```python
from build123d import *

# Parameters (mm, degrees)
SKETCH1_W               = 25.4
SKETCH1_H               = 17.78
BOSS_EXTRUDE1_DEPTH     = 1.6002
CUT_EXTRUDE1_DEPTH      = 16.584695699
CUT_EXTRUDE1_DEPTH_BACK = 16.584695699
SKETCH2_R               = 1.5875
SKETCH3_W               = 15.24
SKETCH3_H               = 2.54
BOSS_EXTRUDE2_DEPTH     = 2.54
SKETCH4_R               = 0.4064
BOSS_EXTRUDE3_DEPTH     = 5.969
LPATTERN1_COUNT         = 6
LPATTERN1_PITCH         = 2.54
MIRROR1_COPY_1_SKETCH_R = 0.4064
MIRROR1_COPY_1_DEPTH    = 5.969
MIRROR1_COPY_2_SKETCH_R = 0.4064
MIRROR1_COPY_2_DEPTH    = 5.969
MIRROR1_COPY_3_SKETCH_R = 0.4064
MIRROR1_COPY_3_DEPTH    = 5.969
MIRROR1_COPY_4_SKETCH_R = 0.4064
MIRROR1_COPY_4_DEPTH    = 5.969
MIRROR1_COPY_5_SKETCH_R = 0.4064
MIRROR1_COPY_5_DEPTH    = 5.969
SKETCH5_W               = 4.445
SKETCH5_H               = 6.35
BOSS_EXTRUDE4_DEPTH     = 3.175


with BuildPart() as part:
    # Sketch1 → Boss-Extrude1 (new body)
    with BuildSketch(Plane(origin=(0, 0, 0), x_dir=(1, 0, 0), z_dir=(0, 1, 0))):
        Rectangle(SKETCH1_W, SKETCH1_H)
    extrude(amount=BOSS_EXTRUDE1_DEPTH)

    # Sketch2 → Cut-Extrude1 (cut, two sides: drawn at the far end of the back side and taken through both)
    with BuildSketch(Plane(origin=(0, 1.6002, 0), x_dir=(1, 0, 0), z_dir=(0, 1, 0)).offset(-CUT_EXTRUDE1_DEPTH_BACK)):
        with Locations(Location((-10.16, 6.35, 0), (0, 0, 270))):
            Circle(SKETCH2_R)
        with Locations(Location((10.16, 6.35, 0), (0, 0, 270))):
            Circle(SKETCH2_R)
        with Locations(Location((10.16, -6.35, 0), (0, 0, 270))):
            Circle(SKETCH2_R)
        with Locations(Location((-10.16, -6.35, 0), (0, 0, 270))):
            Circle(SKETCH2_R)
        with BuildLine():
            Line((-12.7, 6.35), (-12.7, 8.89))
            Line((-12.7, 8.89), (-10.16, 8.89))
            ThreePointArc((-10.16, 8.89), (-11.956051224, 8.146051224), (-12.7, 6.35))
        make_face()
        with BuildLine():
            Line((10.16, 8.89), (12.7, 8.89))
            Line((12.7, 8.89), (12.7, 6.35))
            ThreePointArc((12.7, 6.35), (11.956051224, 8.146051224), (10.16, 8.89))
        make_face()
        with BuildLine():
            Line((10.16, -8.89), (12.7, -8.89))
            Line((12.7, -8.89), (12.7, -6.35))
            ThreePointArc((12.7, -6.35), (11.956051224, -8.146051224), (10.16, -8.89))
        make_face()
        with BuildLine():
            Line((-12.7, -6.35), (-12.7, -8.89))
            Line((-12.7, -8.89), (-10.16, -8.89))
            ThreePointArc((-10.16, -8.89), (-11.956051224, -8.146051224), (-12.7, -6.35))
        make_face()
    extrude(amount=CUT_EXTRUDE1_DEPTH + CUT_EXTRUDE1_DEPTH_BACK, mode=Mode.SUBTRACT)

    # Sketch3 → Boss-Extrude2 (add)
    with BuildSketch(Plane.XZ):
        with Locations((0, 6.35)):
            Rectangle(SKETCH3_W, SKETCH3_H)
    boss_extrude2 = extrude(amount=BOSS_EXTRUDE2_DEPTH)

    # Sketch4 → Boss-Extrude3 (add)
    with BuildSketch(Plane.XZ.offset(2.54)):
        with Locations(Location((-6.35, 6.35, 0), (0, 0, 270))):
            Circle(SKETCH4_R)
    boss_extrude3 = extrude(amount=BOSS_EXTRUDE3_DEPTH)

    # LPattern1: Boss-Extrude3 ×6
    with Locations(*[(i * LPATTERN1_PITCH, 0, 0) for i in range(1, LPATTERN1_COUNT)]):
        add(boss_extrude3)

    # Mirror1: Boss-Extrude2, Boss-Extrude3 across plane
    add(boss_extrude2.mirror(Plane.XY))
    add(boss_extrude3.mirror(Plane.XY))

    # Mirror1 copy 1 sketch → Mirror1 copy 1 (add)
    with BuildSketch(Plane(origin=(2.54, -2.54, 0), x_dir=(1, 0, 0), z_dir=(0, -1, 0))):
        with Locations((-6.35, -6.35)):
            Circle(MIRROR1_COPY_1_SKETCH_R)
    extrude(amount=MIRROR1_COPY_1_DEPTH)

    # Mirror1 copy 2 sketch → Mirror1 copy 2 (add)
    with BuildSketch(Plane(origin=(5.08, -2.54, 0), x_dir=(1, 0, 0), z_dir=(0, -1, 0))):
        with Locations((-6.35, -6.35)):
            Circle(MIRROR1_COPY_2_SKETCH_R)
    extrude(amount=MIRROR1_COPY_2_DEPTH)

    # Mirror1 copy 3 sketch → Mirror1 copy 3 (add)
    with BuildSketch(Plane(origin=(7.62, -2.54, 0), x_dir=(1, 0, 0), z_dir=(0, -1, 0))):
        with Locations((-6.35, -6.35)):
            Circle(MIRROR1_COPY_3_SKETCH_R)
    extrude(amount=MIRROR1_COPY_3_DEPTH)

    # Mirror1 copy 4 sketch → Mirror1 copy 4 (add)
    with BuildSketch(Plane(origin=(10.16, -2.54, 0), x_dir=(1, 0, 0), z_dir=(0, -1, 0))):
        with Locations((-6.35, -6.35)):
            Circle(MIRROR1_COPY_4_SKETCH_R)
    extrude(amount=MIRROR1_COPY_4_DEPTH)

    # Mirror1 copy 5 sketch → Mirror1 copy 5 (add)
    with BuildSketch(Plane(origin=(12.7, -2.54, 0), x_dir=(1, 0, 0), z_dir=(0, -1, 0))):
        with Locations((-6.35, -6.35)):
            Circle(MIRROR1_COPY_5_SKETCH_R)
    extrude(amount=MIRROR1_COPY_5_DEPTH)

    # Sketch5 → Boss-Extrude4 (add)
    with BuildSketch(Plane(origin=(0, 1.6002, 0), x_dir=(1, 0, 0), z_dir=(0, 1, 0))):
        with Locations((-10.3505, 0)):
            Rectangle(SKETCH5_W, SKETCH5_H)
        with Locations((10.3505, 0)):
            Rectangle(SKETCH5_W, SKETCH5_H)
    extrude(amount=BOSS_EXTRUDE4_DEPTH)


solid = part.part
```
The listing builds one solid part. Answer for the finished solid, in the listing's coordinates (mm). A direction names the side the tool comes from. Give positions to 0.01 mm unless a question says otherwise; leave off trailing zeros. Loops run counter-clockwise (first coordinate to the right, second up) from the corner with the lowest first, then second, coordinate; pieces in that order, holes last. Notation, with made-up numbers: (89, 53.5) - (103, 53.5) arc R15 cw to (103, 71.5) - close; hole circle Ø1 at (73.25, -5). An arc over 180 degrees is marked (long way). Answer as CSV lines item,"result". Start each with the question number.
Item 1: Each of these flat-tipped pins is pushed along its axis until it touches: pin 1 (1 mm diameter, centred on x = 8.5, z = 4, fed in from +Y); pin 2 (1 mm diameter, centred on x = -8, z = 5, fed in from -Y); pin 3 (2.5 mm diameter, centred on y = 4, z = -0.5, fed in from +X). Where does it stop, or does it pass through?
Item 2: A cutting plane is placed at B-B on x = 5.25. Determine the outline of the cut face in (y, z).
Item 3: For faces 4 (the face through (-3.42, -5.48, -6.23)), 5 (the face through (0, -1, -5.08)), 6 (the face through (-8.128, 3, 0)), 7 (the face through (10, 4.775, 0)), 8 (the face through (10, 3, 3.175)), determine the directions among +Z, -Z, +X, -X, +Y, -Y from which every point of the face is accessible in a straight line to the end or side of a thin tool.
Item 4: A cutting plane is placed at A-A on y = -5. Count the separate pieces of the cut face and the enclosed holes in it, then the cut area to 3 significant figures.
Item 5: A cutting plane is placed at D-D on x = -3.81. Determine the outline of the cut face in (y, z).
Item 6: A cutting plane is placed at C-C on z = 2.5. Determine the outline of the cut face in (x, y), then the cut area to 3 significant figures.
Item 7: Find the intervals of material crossed by line 1 (X direction, y = 0.8, z = -6.35); line 2 (Z direction, x = 10.16, y = 0.5); line 3 (Z direction, x = -4.5, y = -2), in increasing order. Write a range as from..to.
Item 8: The mould has two halves that part along Z. Classify faces 1 (the face through (10.637, 0.789, -4.836)), 2 (the face through (-7.62, -1, -6)), 3 (the face through (-10, 3, -3.175)): +Z half, -Z half, draft (parallel to the pull), parting line (faces both ways), or undercut.
Found:
1,pin 1,"stops at y = 1.6"
1,pin 2,"stops at y = -2.54"
1,pin 3,"stops at x = 12.57"
2,outline,"(-2.54, -7.62) - (0, -7.62) - (0, -8.89) - (1.6, -8.89) - (1.6, 8.89) - (0, 8.89) - (0, 7.62) - (-2.54, 7.62) - (-2.54, 5.08) - (0, 5.08) - (0, -5.08) - (-2.54, -5.08) - close"
3,face 4,"-Y"
3,face 5,"+X, -X, -Y"
3,face 6,"+Z, -Z, +Y"
3,face 7,"+Z, -Z, +X, -X, +Y"
3,face 8,"+Z, +X, -X, +Y"
4,separate pieces,"12"
4,enclosed holes,"0"
4,area,"6.23 mm^2"
5,outline,"(-8.51, -6.76) - (-2.54, -6.76) - (-2.54, -7.62) - (0, -7.62) - (0, -8.89) - (1.6, -8.89) - (1.6, 8.89) - (0, 8.89) - (0, 7.62) - (-2.54, 7.62) - (-2.54, 6.76) - (-8.51, 6.76) - (-8.51, 5.94) - (-2.54, 5.94) - (-2.54, 5.08) - (0, 5.08) - (0, -5.08) - (-2.54, -5.08) - (-2.54, -5.94) - (-8.51, -5.94) - close"
6,outline,"(-12.7, 0) - (12.7, 0) - (12.7, 1.6) - (12.57, 1.6) - (12.57, 4.78) - (8.13, 4.78) - (8.13, 1.6) - (-8.13, 1.6) - (-8.13, 4.78) - (-12.57, 4.78) - (-12.57, 1.6) - (-12.7, 1.6) - close"
6,area,"68.9 mm^2"
7,line 1,"x = -12.7..-11.75, -8.57..8.57, 11.75..12.7"
7,line 2,"z = -8.89..-7.94, -4.76..4.76, 7.94..8.89"
7,line 3,"z = -7.62..-5.08, 5.08..7.62"
8,face 1,"undercut"
8,face 2,"draft"
8,face 3,"-Z half"
